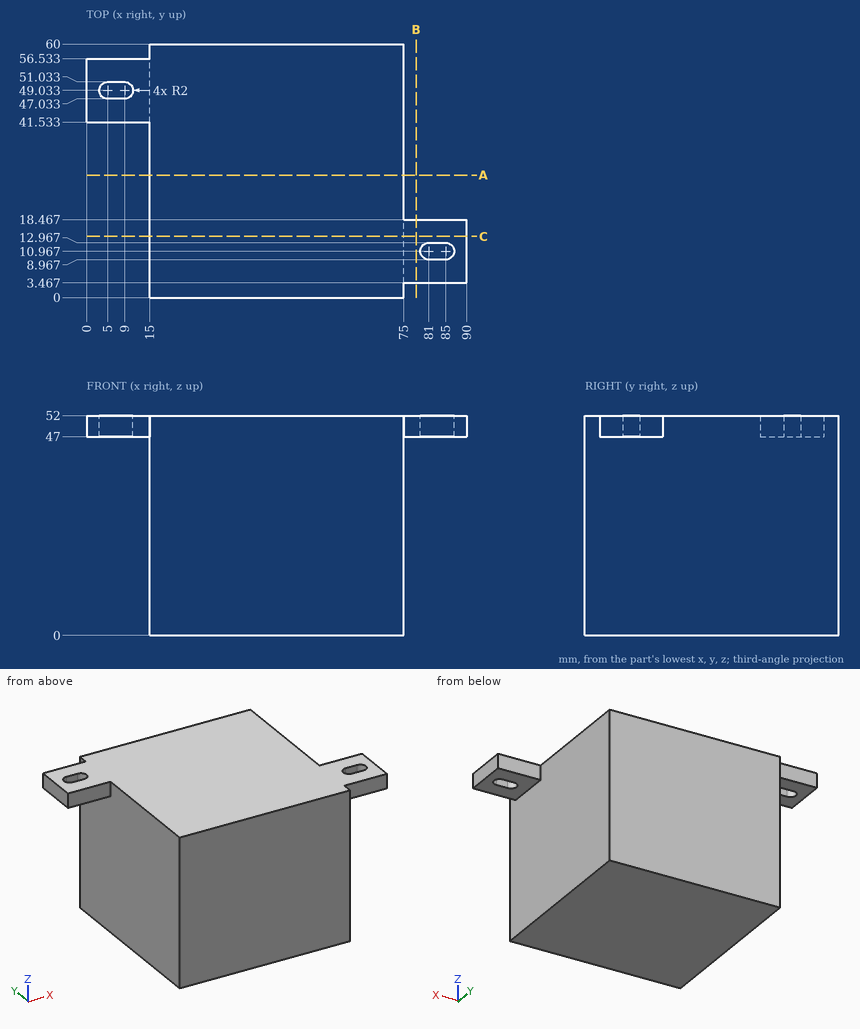
Design review of the part shown in the three views and the two pictorial views. Dimensions are in mm from the part's minimum x, y and z. Give positions to 0.01 mm unless a question says otherwise; leave off trailing zeros. Order: outer loops, then holes, each group sorted by start corner. A loop starts at its lowest first (then second) coordinate and runs counter-clockwise, first axis right, second up. Notation, with made-up numbers: (28, 8.5) -> (69, 8.5) arc R11 ccw to (69, 26.5) -> close; hole circle Ø4 at (51, -7). An arc over 180 degrees is marked (long way). Write each question's results on one line, items separated by ' | '. Start each with the question number.
Q1. Add section C-C on y = 14.5. Give the boundary of the cut face in (x, z).
Q2. Add section A-A on y = 29. Give the boundary of the cut face in (x, z).
Q3. Wall thickness on L1, parallel to X at y = 44, z = 37: over which ranges is the line inside the solid? List them lowest first. Write a range as from..to.
Q4. Add section B-B on x = 78. Give the boundary of the cut face in (y, z).
Q5. For pin 1 (1 mm diameter, centred on x = 70, y = 20.5, fed in from -Z); pin 2 (12 mm diameter, centred on x = 8.5, y = 52, fed in from -Z); pin 3 (3 mm diameter, centred on x = 83.5, z = 48.5, fed in from +Y); pin 4 (5.5 mm diameter, centred on x = 8.5, z = 50, fed in from -Y), all flat-tipped, find the tip position at first contact; note any pin that passes through.
Found:
1) outline: (15, 0) -> (75, 0) -> (75, 47) -> (90, 47) -> (90, 52) -> (15, 52) -> close
2) outline: (15, 0) -> (75, 0) -> (75, 52) -> (15, 52) -> close
3) L1: x = 15..75
4) outline: (3.47, 47) -> (18.47, 47) -> (18.47, 52) -> (3.47, 52) -> close
5) pin 1: stops at z = 0 | pin 2: stops at z = 47 | pin 3: stops at y = 18.47 | pin 4: stops at y = 41.53
